```python
from build123d import *

# Parameters (mm, degrees)
SKETCH1_R           = 14.2875
SKETCH1_R_2         = 2.38125
BOSS_EXTRUDE1_DEPTH = 3.175
SKETCH2_R           = 18.832202279
SKETCH2_R_2         = 14.2875
CUT_EXTRUDE1_DEPTH  = 21.453506729


with BuildPart() as part:
    # Sketch1 → Boss-Extrude1 (new body)
    with BuildSketch(Plane.XY):
        Circle(SKETCH1_R)
        with Locations((0, 7.9375)):
            Circle(SKETCH1_R_2, mode=Mode.SUBTRACT)
        with Locations((0, -7.9375)):
            Circle(SKETCH1_R_2, mode=Mode.SUBTRACT)
    extrude(amount=BOSS_EXTRUDE1_DEPTH)

    # Sketch2 → Cut-Extrude1 (cut, through all)
    # profile 1 of 5: a face of its own
    with BuildSketch(Plane.XY.offset(3.175)):
        Circle(SKETCH2_R)
        Circle(SKETCH2_R_2, mode=Mode.SUBTRACT)
    # profile 2 of 5: a face of its own
    with BuildSketch(Plane.XY.offset(3.175)):
        with BuildLine():
            ThreePointArc((4.340071127, 12.572829828), (7.875864823, 9.874463076), (11.879762203, 7.9375))
            ThreePointArc((11.879762203, 7.9375), (6.735192091, 12.600390619), (0, 14.2875))
            ThreePointArc((0, 14.2875), (2.333254764, 13.843295645), (4.340071127, 12.572829828))
        make_face()
    # profile 3 of 5: a face of its own
    with BuildSketch(Plane.XY.offset(3.175)):
        with BuildLine():
            ThreePointArc((7.3e-08, -14.2875), (6.735192123, -12.600390602), (11.879762203, -7.9375))
            ThreePointArc((11.879762203, -7.9375), (7.875864823, -9.874463076), (4.340071127, -12.572829828))
            ThreePointArc((4.340071127, -12.572829828), (2.333254798, -13.843295632), (7.3e-08, -14.2875))
        make_face()
    # profile 4 of 5: a face of its own
    with BuildSketch(Plane.XY.offset(3.175)):
        with BuildLine():
            ThreePointArc((-11.879762203, -7.9375), (-6.735192059, -12.600390636), (7.3e-08, -14.2875))
            ThreePointArc((7.3e-08, -14.2875), (-2.33325473, -13.843295659), (-4.340071127, -12.572829828))
            ThreePointArc((-4.340071127, -12.572829828), (-7.875864823, -9.874463076), (-11.879762203, -7.9375))
        make_face()
    # profile 5 of 5: a face of its own
    with BuildSketch(Plane.XY.offset(3.175)):
        with BuildLine():
            ThreePointArc((-4.340071127, 12.572829828), (-2.333254764, 13.843295645), (0, 14.2875))
            ThreePointArc((0, 14.2875), (-6.735192091, 12.600390619), (-11.879762203, 7.9375))
            ThreePointArc((-11.879762203, 7.9375), (-7.875864823, 9.874463076), (-4.340071127, 12.572829828))
        make_face()
    extrude(amount=-CUT_EXTRUDE1_DEPTH, mode=Mode.SUBTRACT)


solid = part.part
```
Design review of the part built by this model. Coordinates are the model's own, in mm. Coordinates: 2 decimals unless noted, no trailing zeros. Write each loop counter-clockwise with the first axis right and the second up, starting at its lowest first coordinate (ties: lowest second). Pieces come first, ordered by that corner, then holes.
1) Mouldability with a two-part tool opening along X and no side actions: class faces 1 (the cylindrical face through (-0.516, 5.613, 1.565)), 2 (the cylindrical face through (7.93, -9.84, 1.61)), 3 (the cylindrical face through (-0.52, -10.26, 1.57)), 4 (the cylindrical face through (-7.93, 9.84, 1.61)) as +X half, -X half, draft (parallel to the pull), parting line (faces both ways), or undercut.
2) Insertion check: pin 1 (2 mm diameter, centred on x = -2.5, y = -7, fed in from -Z). The pin has a flat end and moves straight along its axis. Give the tip position at first contact, or say it passes through.
3) Add section C-C (x = -1.25). Write out the cut boundary in (y, z) (3 decimals), plus the area to 3 significant figures.
4) To check wall thickness, follow L1, parallel to X at y = -6.5, z = 2.2; L2, parallel to Y at x = -0.25, z = 0.4; L3, parallel to X at y = 6.75, z = 2. State the ranges of each line that lie inside material, in increasing order.
5) Add section A-A (y = 7). Write out the cut boundary in (x, z) (3 decimals), plus the area to 3 significant figures.
6) Add section B-B (z = 2.2). State how many separate pieces and enclosed holes the cut face has, plus the area to 3 significant figures.
7) Add section D-D (x = 8.75). Write out the cut boundary in (y, z) (3 decimals).
Check result:
1. face 1: undercut
1. face 2: +X half
1. face 3: undercut
1. face 4: -X half
2. pin 1: stops at z = 0
3. outline: (-14.163, 0) - (-9.964, 0) - (-9.964, 3.175) - (-14.163, 3.175) - close; (-5.911, 0) - (5.911, 0) - (5.911, 3.175) - (-5.911, 3.175) - close; (9.964, 0) - (14.163, 0) - (14.163, 3.175) - (9.964, 3.175) - close
3. area: 64.2 mm2
4. L1: x = -12.72 to -1.9, 1.9 to 12.72
4. L2: y = -14.28 to -10.31, -5.57 to 5.57, 10.31 to 14.28
4. L3: x = -12.59 to -2.06, 2.06 to 12.59
5. outline: (-12.455, 0) - (-2.189, 0) - (-2.189, 3.175) - (-12.455, 3.175) - close; (2.189, 0) - (12.455, 0) - (12.455, 3.175) - (2.189, 3.175) - close
5. area: 65.2 mm2
6. separate pieces: 1
6. enclosed holes: 2
6. area: 554 mm2
7. outline: (-9.364, 0) - (9.364, 0) - (9.364, 3.175) - (-9.364, 3.175) - close
